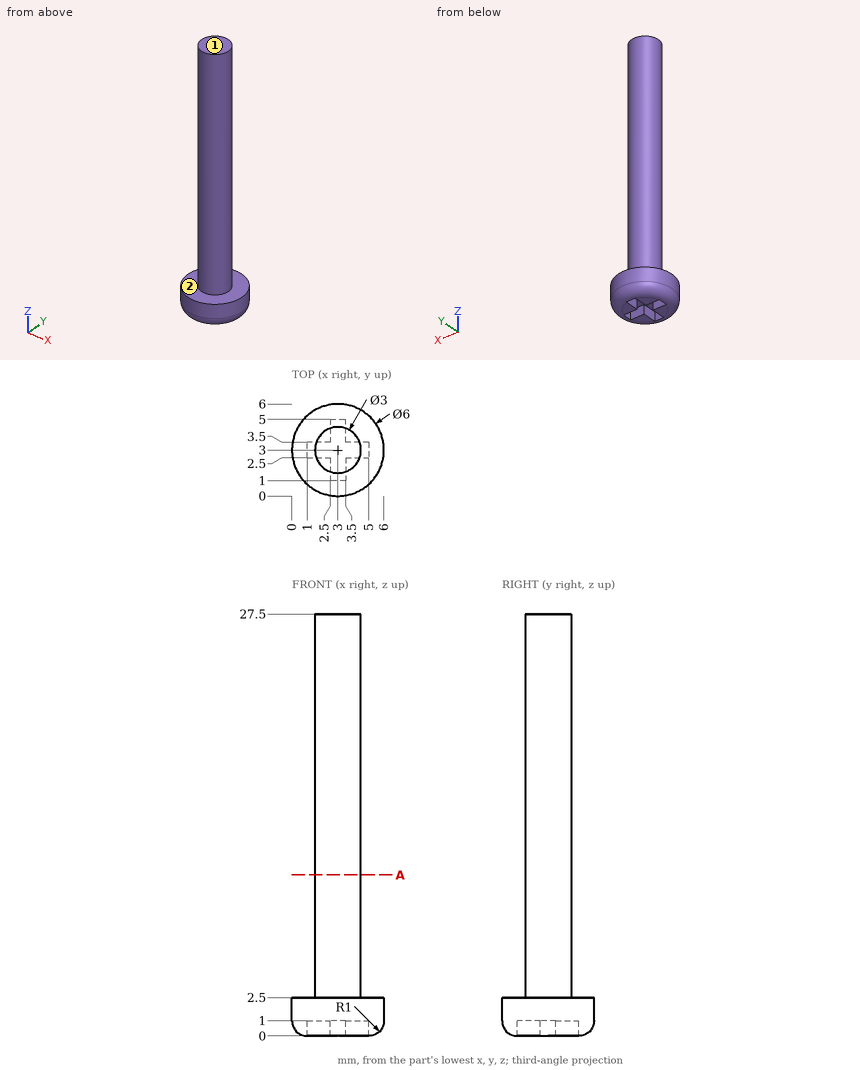
Geometry: see drawing. Coordinates: mm, zero at the bounding-box minimum. A direction names the side the tool comes from. Coordinates: 2 decimals unless noted, no trailing zeros. Order: outer loops, then holes, each group sorted by start corner. A loop starts at its lowest first (then second) coordinate and runs counter-clockwise, first axis right, second up. Notation, with made-up numbers: (43, -1.5) - (66, -1.5) arc R34 ccw to (66, 28.5) - close; hole circle Ø8 at (43.5, 27.5). An arc over 180 degrees is marked (long way). Return JSON: item names as keys, results as strings.
Q1. Ray query, probe 1 along Z at (x, y) = (2, 3.25); probe 2 along Y at (x, z) = (3.5, 4); probe 3 along Z at (x, y) = (1, 2). Return the intervals inside material, ascending.
The answers:
{"probe 1": "z = 1 to 27.5", "probe 2": "y = 1.59 to 4.41", "probe 3": "z = 0.03 to 2.5"}
Q2. Access query for the marked faces 1 and 2. Directions: +Z, -Z, +X, -X, +Y, -Y. A direction counts if a zero-diameter tool reaches every point of the face in a straight line with its end or side. Return the directions, or none.
The answers:
{"face 1": "+Z, +X, -X, +Y, -Y", "face 2": "+Z"}
Q3. Cut plane A-A (z = 10.5). Return loops of the section in (x, y), then the cut area to 3 significant figures.
The answers:
{"outline": "circle Ø3 at (3, 3)", "area": "7.07 mm2"}
Q4. First-contact query: pin 1 (1.1 mm diameter, centred on y = 1.5, z = 0.5, fed in from +X); pin 2 (0.5 mm diameter, centred on x = 4, z = 0.5, fed in from -Y); pin 3 (0.8 mm diameter, centred on y = 4, z = 0.5, fed in from +X). Flat tips, straight axial feed; report the tip coordinate or a pass-through.
The answers:
{"pin 1": "stops at x = 5.79", "pin 2": "stops at y = 0.17", "pin 3": "stops at x = 5.89"}
